Could you check a few things on this model? Use its own coordinates, in mm. Give positions to 0.01 mm unless a question says otherwise; leave off trailing zeros. Write each loop counter-clockwise with the first axis right and the second up, starting at its lowest first coordinate (ties: lowest second). Pieces come first, ordered by that corner, then holes. Notation, with made-up numbers: (38.25, 80.5) - (64.25, 80.5) arc R36 cw to (64.25, 116.5) - close; hole circle Ø7 at (81, 29). An arc over 180 degrees is marked (long way). Answer in a Markdown table with one row per item.
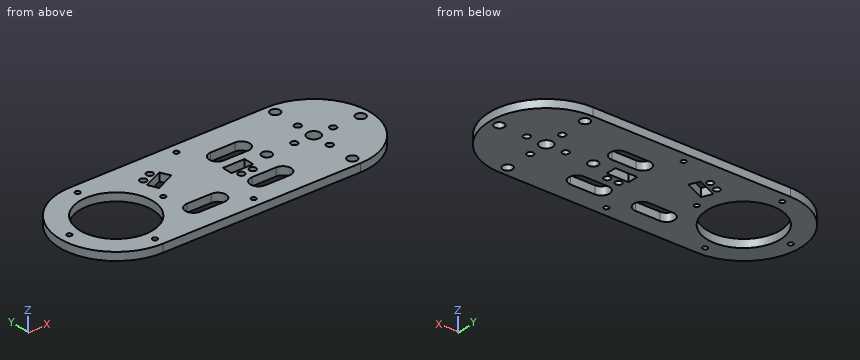
from build123d import *

# Parameters (mm, degrees)
SKETCH1_R           = 4
SKETCH1_R_2         = 22.5
SKETCH1_R_3         = 1.5
SKETCH1_R_4         = 3
SKETCH1_R_5         = 2
SKETCH1_W           = 13.5
SKETCH1_H           = 6.5
BOSS_EXTRUDE1_DEPTH = 5


with BuildPart() as part:
    # Sketch1 → Boss-Extrude1 (new body)
    with BuildSketch(Plane.XY):
        with BuildLine():
            Line((61, -35), (-61, -35))
            ThreePointArc((-61, -35), (-96, 0), (-61, 35))
            Line((-61, 35), (61, 35))
            ThreePointArc((61, 35), (96, 0), (61, -35))
        make_face()
        with Locations((61, 0)):
            Circle(SKETCH1_R, mode=Mode.SUBTRACT)
        with Locations((-61, 0)):
            Circle(SKETCH1_R_2, mode=Mode.SUBTRACT)
        with Locations((-61, -29)):
            Circle(SKETCH1_R_3, mode=Mode.SUBTRACT)
        with Locations((-61, 29)):
            Circle(SKETCH1_R_3, mode=Mode.SUBTRACT)
        with Locations((61, 29)):
            Circle(SKETCH1_R_4, mode=Mode.SUBTRACT)
        with Locations((61, -29)):
            Circle(SKETCH1_R_4, mode=Mode.SUBTRACT)
        with Locations((0, -29)):
            Circle(SKETCH1_R_3, mode=Mode.SUBTRACT)
        with Locations((0, 29)):
            Circle(SKETCH1_R_3, mode=Mode.SUBTRACT)
        with Locations((-90, 0)):
            Circle(SKETCH1_R_3, mode=Mode.SUBTRACT)
        with Locations((-32, 0)):
            Circle(SKETCH1_R_3, mode=Mode.SUBTRACT)
        with Locations((90, 0)):
            Circle(SKETCH1_R_4, mode=Mode.SUBTRACT)
        with Locations((32, 0)):
            Circle(SKETCH1_R_4, mode=Mode.SUBTRACT)
        with Locations((61, 12)):
            Circle(SKETCH1_R_5, mode=Mode.SUBTRACT)
        with Locations((61, -12)):
            Circle(SKETCH1_R_5, mode=Mode.SUBTRACT)
        with Locations((49, 0)):
            Circle(SKETCH1_R_5, mode=Mode.SUBTRACT)
        with Locations((73, 0)):
            Circle(SKETCH1_R_5, mode=Mode.SUBTRACT)
        with Locations((10.75, -6.75)):
            Circle(SKETCH1_R_5, mode=Mode.SUBTRACT)
        with Locations((17.75, -6.75)):
            Circle(SKETCH1_R_5, mode=Mode.SUBTRACT)
        with Locations((-23.054905042, 20.964824554)):
            Circle(SKETCH1_R_5, mode=Mode.SUBTRACT)
        with Locations((-29.435230641, 18.085337577)):
            Circle(SKETCH1_R_5, mode=Mode.SUBTRACT)
        with Locations((14.25, 0)):
            Rectangle(SKETCH1_W, SKETCH1_H, mode=Mode.SUBTRACT)
        with BuildLine():
            Line((-27.66, -12.5), (-12.66, -12.5))
            ThreePointArc((-12.66, -12.5), (-7.66, -17.5), (-12.66, -22.5))
            Line((-12.66, -22.5), (-27.66, -22.5))
            ThreePointArc((-27.66, -22.5), (-32.66, -17.5), (-27.66, -12.5))
        make_face(mode=Mode.SUBTRACT)
        with BuildLine():
            Line((12.5, -12.5), (27.5, -12.5))
            ThreePointArc((27.5, -12.5), (32.5, -17.5), (27.5, -22.5))
            Line((27.5, -22.5), (12.5, -22.5))
            ThreePointArc((12.5, -22.5), (7.5, -17.5), (12.5, -12.5))
        make_face(mode=Mode.SUBTRACT)
        with BuildLine():
            Line((12.5, 18.47), (27.5, 18.47))
            ThreePointArc((27.5, 18.47), (32.5, 13.47), (27.5, 8.47))
            Line((27.5, 8.47), (12.5, 8.47))
            ThreePointArc((12.5, 8.47), (7.5, 13.47), (12.5, 18.47))
        make_face(mode=Mode.SUBTRACT)
        Polygon((-30.95778118, 13.55827011), (-28.283971844, 7.633682054), (-15.979058189, 13.186978367), (-18.652867525, 19.111566423), align=None, mode=Mode.SUBTRACT)
    extrude(amount=BOSS_EXTRUDE1_DEPTH)


solid = part.part
1) Imagine slicing it at B-B (y = -18). List the corners of the cut face in (x, z) for me, then the cut area to 3 significant figures.
Check values:
| item | result |
|---|---|
| outline | (-91.02, 0) - (-74.5, 0) - (-74.5, 5) - (-91.02, 5) - close; (-47.5, 0) - (-32.63, 0) - (-32.63, 5) - (-47.5, 5) - close; (-7.69, 0) - (7.53, 0) - (7.53, 5) - (-7.69, 5) - close; (32.47, 0) - (91.02, 0) - (91.02, 5) - (32.47, 5) - close |
| area | 526 mm2 |
2) Imagine slicing it at D-D (z = 1.6). State how many separate pieces and enclosed holes the cut face has, then the cut area to 3 significant figures.
Check values:
| item | result |
|---|---|
| separate pieces | 1 |
| enclosed holes | 25 |
| area | 9,630 mm2 |
3) Imagine slicing it at C-C (y = -6.75). List the corners of the cut face in (x, z) for me, then the cut area to 3 significant figures.
Check values:
| item | result |
|---|---|
| outline | (-95.34, 0) - (-82.46, 0) - (-82.46, 5) - (-95.34, 5) - close; (-39.54, 0) - (8.75, 0) - (8.75, 5) - (-39.54, 5) - close; (12.75, 0) - (15.75, 0) - (15.75, 5) - (12.75, 5) - close; (19.75, 0) - (95.34, 0) - (95.34, 5) - (19.75, 5) - close |
| area | 699 mm2 |
4) Imagine slicing it at A-A (x = 73). List the corners of the cut face in (y, z) for me.
Check values:
| item | result |
|---|---|
| outline | (-32.88, 0) - (-2, 0) - (-2, 5) - (-32.88, 5) - close; (2, 0) - (32.88, 0) - (32.88, 5) - (2, 5) - close |
5) If I drill on line 1 (Y direction, x = 61, z = 2.5); line 2 (Y direction, x = 0, z = 4.05); line 3 (Y direction, x = -30, z = 3.5), over which ranges is the centre line in solid material (lowest first)?
Check values:
| item | result |
|---|---|
| line 1 | y = -35 to -32, -26 to -14, -10 to -4, 4 to 10, 14 to 26, 32 to 35 |
| line 2 | y = -35 to -30.5, -27.5 to 27.5, 30.5 to 35 |
| line 3 | y = -35 to -21.92, -13.08 to 11.44, 13.99 to 16.17, 20 to 35 |
